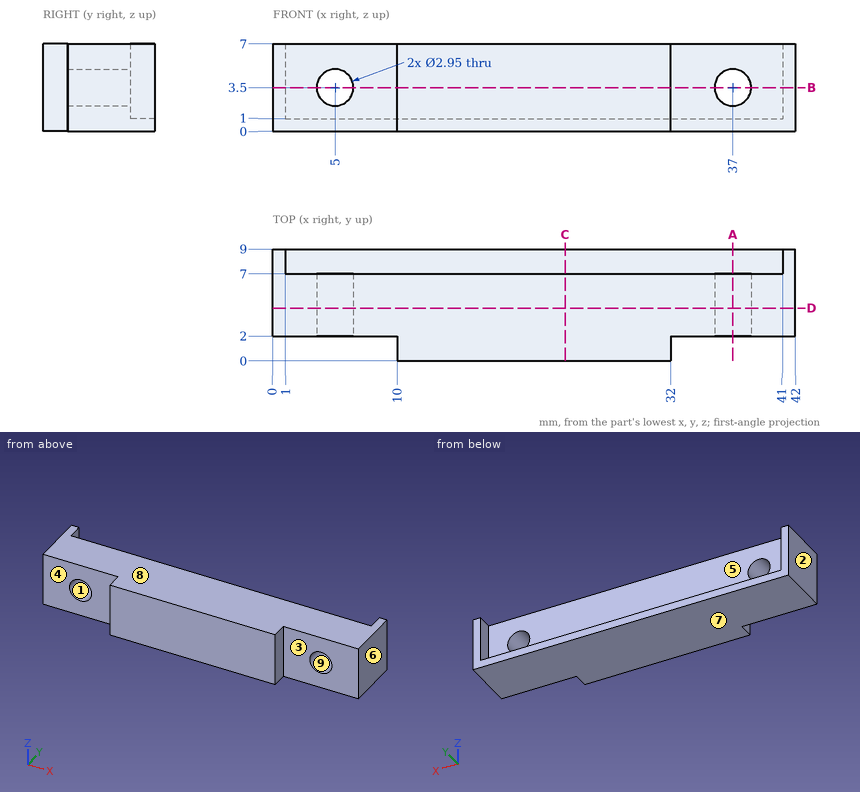
Geometry check sheet. Reference: drawing and pictorial views, mm from the part's lowest x, y, z. A direction names the side the tool comes from. Coordinates: 2 decimals unless noted, no trailing zeros. Order: outer loops, then holes, each group sorted by start corner. A loop starts at its lowest first (then second) coordinate and runs counter-clockwise, first axis right, second up. Notation, with made-up numbers: (-36, 10.25) - (8, 10.25) arc R26 ccw to (8, 46.25) - close; hole circle Ø6 at (-22.5, 15.5). An arc over 180 degrees is marked (long way). One line per item, written item: value.
(1) Sectioned sample at D-D (y = 4.25). Enter the section's corners in (x, z) (3 decimals).
Data:
outline: (0, 0) - (42, 0) - (42, 7) - (0, 7) - close; hole circle Ø2.95 at (5, 3.5); hole circle Ø2.95 at (37, 3.5)
(2) Sectioned sample at B-B (z = 3.5). Enter the section's corners in (x, y) (3 decimals), and give its area (4 significant figures).
Data:
outline: (0, 2) - (3.525, 2) - (3.525, 7) - (1, 7) - (1, 9) - (0, 9) - close; (6.475, 2) - (10, 2) - (10, 0) - (32, 0) - (32, 2) - (35.525, 2) - (35.525, 7) - (6.475, 7) - close; (38.475, 2) - (42, 2) - (42, 9) - (41, 9) - (41, 7) - (38.475, 7) - close
area: 228.5 mm^2
(3) Sectioned sample at C-C (x = 23.5). Enter the section's corners in (y, z).
Data:
outline: (0, 0) - (9, 0) - (9, 1) - (7, 1) - (7, 7) - (0, 7) - close
(4) Sectioned sample at A-A (x = 37). Enter the section's corners in (y, z) (3 decimals), and give its area (4 significant figures).
Data:
outline: (2, 0) - (9, 0) - (9, 1) - (7, 1) - (7, 2.025) - (2, 2.025) - close; (2, 4.975) - (7, 4.975) - (7, 7) - (2, 7) - close
area: 22.25 mm^2
(5) Thickness scan on probe 1 along X at (y, z) = (5.6, 3.5) (3 decimals); probe 2 along Z at (x, y) = (37, 4.7) (3 decimals); probe 3 along X at (y, z) = (8.25, 5.5). Record the ranges inside material, lowest first. Write a range as from..to.
Data:
probe 1: x = 0..3.525, 6.475..35.525, 38.475..42
probe 2: z = 0..2.025, 4.975..7
probe 3: x = 0..1, 41..42
(6) Release check for a two-part mould opening along Z. For the marked faces 6, 7, 8 and 9 record: +Z half, -Z half, draft (parallel to the pull), parting line (faces both ways), or undercut.
Data:
face 6: draft
face 7: -Z half
face 8: +Z half
face 9: undercut
(7) Depth check by flat-ended pin: pin 1 Ø0.6 at (y, z) = (1, 4.5) entering from +X; pin 2 Ø3.5 at (x, z) = (5, 3.5) entering from -Y; pin 3 Ø1.5 at (x, z) = (29.5, 2.5) entering from +Y. Enter the tip coordinate at first touch or a pass-through.
Data:
pin 1: stops at x = 32
pin 2: stops at y = 2
pin 3: stops at y = 7
(8) Access from +Z, -Z, +X, -X, +Y, -Y to the whole of each face (thin tool, end or side, straight path). Record for the marked faces 1, 2, 3, 4 and 5.
Data:
face 1: +Y, -Y
face 2: +Z, -Z, -X, +Y, -Y
face 3: +Z, -Z, +X, -Y
face 4: +Z, -Z, -X, -Y
face 5: +Z, +Y
